Here's how the part is built. I have some questions about the finished solid (model axes, mm). A direction names the side the tool comes from. Round coordinates to 2 decimals unless told otherwise and drop trailing zeros. Loops run counter-clockwise (first coordinate to the right, second up) from the corner with the lowest first, then second, coordinate; pieces in that order, holes last. Notation, with made-up numbers: M 52.25,70.5 L 70.25,70.5 A9 cw 70.25,76.5 Z; hole C 24.25,57.5 d11. An arc over 180 degrees is marked long. Answer as a JSON object with one key per item and string values.
from build123d import *

# Parameters (mm, degrees)
ESQUISSE1_W             = 20
ESQUISSE1_H             = 22.5
ESQUISSE1_R             = 2.75
BOSS_EXTRU_1_DEPTH      = 5
BOSS_EXTRU_2_DEPTH      = 15
ENL_V_MAT_EXTRU_1_REACH = 66.95
ESQUISSE3_R             = 1


with BuildPart() as part:
    # Esquisse1 → Boss.-Extru.1 (new body)
    with BuildSketch(Plane.XY):
        with Locations((-27.825146679, -3.282272289)):
            Rectangle(ESQUISSE1_W, ESQUISSE1_H)
        with Locations((-27.825146679, 2.217727711)):
            Circle(ESQUISSE1_R, mode=Mode.SUBTRACT)
        with Locations((-27.825146679, -8.782272289)):
            Circle(ESQUISSE1_R, mode=Mode.SUBTRACT)
    extrude(amount=BOSS_EXTRU_1_DEPTH)

    # Esquisse4 → Boss.-Extru.2 (add)
    with BuildSketch(Plane.ZY.offset(37.825146679)):
        Polygon((5, -14.532272289), (-30, -14.532272289), (-30, -39.532272289), (-25, -39.532272289), (-25, -19.532272289), (5, -19.532272289), align=None)
    extrude(amount=-BOSS_EXTRU_2_DEPTH)

    # Esquisse3 → Enlèv. mat.-Extru.1 (cut, up to next)
    with BuildSketch(Plane.XY.offset(-30), mode=Mode.PRIVATE) as enl_v_mat_extru_1_sk1:
        with Locations((-25.575146679, -34.532272289)):
            Circle(ESQUISSE3_R)
    enl_v_mat_extru_1_tool1 = extrude(enl_v_mat_extru_1_sk1.sketch, amount=ENL_V_MAT_EXTRU_1_REACH, mode=Mode.PRIVATE) & part.part
    # Esquisse3 → Enlèv. mat.-Extru.1 (cut, up to next)
    with BuildSketch(Plane.XY.offset(-30), mode=Mode.PRIVATE) as enl_v_mat_extru_1_sk2:
        with Locations((-35.075146679, -34.532272289)):
            Circle(ESQUISSE3_R)
    enl_v_mat_extru_1_tool2 = extrude(enl_v_mat_extru_1_sk2.sketch, amount=ENL_V_MAT_EXTRU_1_REACH, mode=Mode.PRIVATE) & part.part
    add(enl_v_mat_extru_1_tool1.solids().sort_by_distance((-25.575147, -34.532272, -30))[0], mode=Mode.SUBTRACT)
    add(enl_v_mat_extru_1_tool2.solids().sort_by_distance((-35.075147, -34.532272, -30))[0], mode=Mode.SUBTRACT)


solid = part.part
Item 1: I want a section at C-C, the plane z = 0.5. Please give me the cut outline in (x, y), then the cut area to 3 significant figures.
Resolved:
{"outline": "M -37.83,-19.53 L -22.83,-19.53 L -22.83,-14.53 L -17.83,-14.53 L -17.83,7.97 L -37.83,7.97 Z; hole C -27.83,-8.78 d5.5; hole C -27.83,2.22 d5.5", "area": "477 mm²"}
Item 2: If we mould it in two halves opening along Y, with no side actions, what happens to faces 6 (the face through (-30, -39.532, -28)), 7 (the face through (-28, 7.968, 2)), 8 (the face through (-35.21, -33.54, -27.54)), 9 (the face through (-17.825, -3, 2))? For each: pulls with the +Y half, pulls with the -Y half, needs draft (parallel to the pull), parting line crosses it, or undercut.
Resolved:
{"face 6": "pulls with the -Y half", "face 7": "pulls with the +Y half", "face 8": "undercut", "face 9": "needs draft"}
Item 3: I want a section at A-A, the plane y = 3. Please give me the cut outline in (x, z).
Resolved:
{"outline": "M -37.83,0 L -30.46,0 L -30.46,5 L -37.83,5 Z; M -25.19,0 L -17.83,0 L -17.83,5 L -25.19,5 Z"}
Item 4: I want a section at D-D, the plane x = -26. Please give me the cut outline in (y, z).
Resolved:
{"outline": "M -39.53,-30 L -35.44,-30 L -35.44,-25 L -39.53,-25 Z; M -33.63,-30 L -14.53,-30 L -14.53,0 L -10.84,0 L -10.84,5 L -19.53,5 L -19.53,-25 L -33.63,-25 Z; M -6.73,0 L 0.16,0 L 0.16,5 L -6.73,5 Z; M 4.27,0 L 7.97,0 L 7.97,5 L 4.27,5 Z"}
Item 5: I want a section at B-B, the plane x = -29.75. Please give me the cut outline in (y, z), then the cut area to 3 significant figures.
Resolved:
{"outline": "M -39.53,-30 L -14.53,-30 L -14.53,0 L -10.75,0 L -10.75,5 L -19.53,5 L -19.53,-25 L -39.53,-25 Z; M -6.82,0 L 0.25,0 L 0.25,5 L -6.82,5 Z; M 4.18,0 L 7.97,0 L 7.97,5 L 4.18,5 Z", "area": "348 mm²"}
Item 6: I'm going to push flat-ended pins straight in: pin 1 Ø2.5 at (x, z) = (-20.5, 3) entering from -Y; pin 2 Ø3 at (x, y) = (-25.58, -34.53) entering from +Z; pin 3 Ø6 at (x, y) = (-21.5, 0.5) entering from -Z. Where does each tip first touch, or does it pass through?
Resolved:
{"pin 1": "y = -14.53", "pin 2": "z = -25", "pin 3": "z = 0"}
Item 7: On a 3-axis mill with a long thin cutter (end or side, diameter ignored), from which of +Z, -Z, +X, -X, +Y, -Y can I reach the whole of each face in a straight line? I mean faces 1 (the face through (-30.572, 2.339, 2.465)), 2 (the face through (-20, -14.532, 2)), 3 (the face through (-30, -14.532, -15)), 4 (the face through (-30, -6, 5)), 5 (the face through (-30, -30, -25)). Say none if no direction works.
Resolved:
{"face 1": "+Z, -Z", "face 2": "+Z, -Z, +X, -Y", "face 3": "-Z, +X, -X, +Y", "face 4": "+Z, +X, -X, +Y, -Y", "face 5": "+Z, +X, -X, -Y"}
Item 8: Please list where these lines run through material, in increasing order: probe 1 along Z at (x, y) = (-33.5, 2); probe 2 along Y at (x, z) = (-29.5, -7.5); probe 3 along X at (y, z) = (-27.5, -27). Write a range as from..to.
Resolved:
{"probe 1": "0..5", "probe 2": "-19.53..-14.53", "probe 3": "-37.83..-22.83"}
